```python
from build123d import *

# Parameters (mm, degrees)
CROQUIS1_R              = 17.5
CROQUIS1_R_2            = 1
SALIENTE_EXTRUIR1_DEPTH = 3
SALIENTE_EXTRUIR2_DEPTH = 8
CORTAR_EXTRUIR1_REACH   = 34.974
CROQUIS3_R              = 1.75


with BuildPart() as part:
    # Croquis1 → Saliente-Extruir1 (new body)
    with BuildSketch(Plane.XY):
        Circle(CROQUIS1_R)
        with Locations((0, 9.5)):
            Circle(CROQUIS1_R_2, mode=Mode.SUBTRACT)
        with Locations((9.5, 0)):
            Circle(CROQUIS1_R_2, mode=Mode.SUBTRACT)
        with Locations((0, -9.5)):
            Circle(CROQUIS1_R_2, mode=Mode.SUBTRACT)
        with Locations((-9.5, 0)):
            Circle(CROQUIS1_R_2, mode=Mode.SUBTRACT)
    extrude(amount=SALIENTE_EXTRUIR1_DEPTH)

    # Croquis2 → Saliente-Extruir2 (add)
    with BuildSketch(Plane.XY.offset(3)):
        Polygon((1.993579006, 7.881819991), (-5.829066837, 5.667400059), (-7.822645843, -2.214419931), (-1.993579006, -7.881819991), (5.829066837, -5.667400059), (7.822645843, 2.214419931), align=None)
    extrude(amount=SALIENTE_EXTRUIR2_DEPTH)

    # Croquis3 → Cortar-Extruir1 (cut, up to next)
    with BuildSketch(Plane(origin=(1.917743915, -6.774610025, 0), x_dir=(0.9621911038516526, 0.27237525524308964, 0), z_dir=(0.27237525524308964, -0.9621911038516526, 0)), mode=Mode.PRIVATE) as cortar_extruir1_sk1:
        with Locations((0, 7)):
            Circle(CROQUIS3_R)
    cortar_extruir1_tool1 = extrude(cortar_extruir1_sk1.sketch, amount=-CORTAR_EXTRUIR1_REACH, mode=Mode.PRIVATE) & part.part
    add(cortar_extruir1_tool1.solids().sort_by_distance((1.917744, -6.77461, 7))[0], mode=Mode.SUBTRACT)


solid = part.part
```
The listing builds one solid part. Answer for the finished solid, in the listing's coordinates (mm). A direction names the side the tool comes from. Give positions to 0.01 mm unless a question says otherwise; leave off trailing zeros. Loops run counter-clockwise (first coordinate to the right, second up) from the corner with the lowest first, then second, coordinate; pieces in that order, holes last. Notation, with made-up numbers: M 31,25 L 89,25 A22 cw 89,43 Z; hole C -40,12 d7. An arc over 180 degrees is marked long. One line per item, written item: value.
1. Section D-D on z = 3.75 is taken. Determine the outline of the cut face in (x, y), plus the area to 3 significant figures.
Found:
outline: M -7.82,-2.21 L -1.99,-7.88 L 5.83,-5.67 L 7.82,2.21 L 1.99,7.88 L -5.83,5.67 Z
area: 172 mm^2
2. Find the intervals of material crossed by probe 1 along Y at (x, z) = (0, 2.05); probe 2 along Z at (x, y) = (-9, 5); probe 3 along Y at (x, z) = (9.5, 1.75), in increasing order.
Found:
probe 1: -17.5 to -10.5, -8.5 to 8.5, 10.5 to 17.5
probe 2: 0 to 3
probe 3: -14.7 to -1, 1 to 14.7
3. For a pull along Y with two mould halves and no side action, classify faces 4 (the face through (-6.812, 1.782, 6.944)), 5 (the face through (0, -8, 3)), 6 (the face through (-10.3, -0.6, 1.5)) as pulls with the +Y half, pulls with the -Y half, needs draft (parallel to the pull), parting line crosses it, or undercut.
Found:
face 4: pulls with the +Y half
face 5: needs draft
face 6: undercut
4. Section C-C on z = 5.75 is taken. Determine the outline of the cut face in (x, y), plus the area to 3 significant figures.
Found:
outline: M -7.82,-2.21 L -1.99,-7.88 L 0.74,-7.11 L -3.1,6.44 L -5.83,5.67 Z; M -0.74,7.11 L 3.1,-6.44 L 5.83,-5.67 L 7.82,2.21 L 1.99,7.88 Z
area: 137 mm^2
5. Section A-A on y = -9.5 is taken. Determine the outline of the cut face in (x, z).
Found:
outline: M -14.7,0 L -1,0 L -1,3 L -14.7,3 Z; M 1,0 L 14.7,0 L 14.7,3 L 1,3 Z
6. Each of these flat-tipped pins is pushed along its axis until it touches: P1, Ø1.6, axis at x = 0, y = -9.5, coming from the +Z side; P2, Ø6, axis at x = 6.5, z = 6.5, coming from the +Y side; P3, Ø6, axis at x = 2.5, z = 7, coming from the -Y side; P4, Ø3, axis at x = 9.5, y = 0, coming from the +Z side. Where does it stop, or does it pass through?
Found:
P1: through
P2: y = 6.42
P3: y = -7.46
P4: z = 3
7. For faces 1 (the face through (-4.95, -5.01, 6.94)), 2 (the face through (-2.732, 6.544, 5.166)), 3 (the face through (6.812, -1.782, 6.944)), determine the directions among +Z, -Z, +X, -X, +Y, -Y from which every point of the face is accessible in a straight line to the end or side of a thin tool.
Found:
face 1: +Z, -X, -Y
face 2: +Z, -X, +Y
face 3: +Z, +X, -Y
